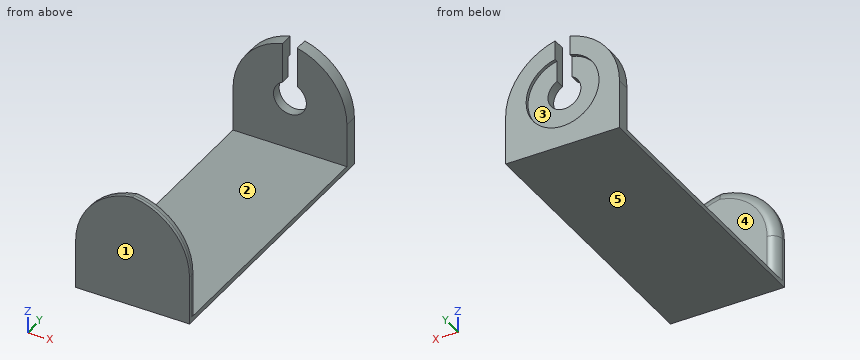
from build123d import *

# Parameters (mm, degrees)
F1_DEPTH    = 17.5
F2_T1_DEPTH = 104
F2_T3_DEPTH = 104
F4_DEPTH    = 1
F5_DEPTH    = 25
F6_R        = 3


# Not quite as in the source:
# - a fillet or chamfer that OpenCascade refuses, or shapes differently, is made with other operations: its cross-section is extruded or revolved along the edge and cut away or added


with BuildPart() as f1:
    # F0 (on Right) → F1 (new body, symmetric)
    with BuildSketch(Plane.YZ):
        Polygon((-44, 35), (-44, 0), (44, 0), (44, 35), (40, 35), (40, 1.5), (-40, 1.5), (-40, 35), align=None)
    extrude(amount=F1_DEPTH, both=True)

    # F2: fillet of radius 20 on 4 edges, made by hand

    # F2_s2 → F2_t1 (cut)
    with BuildSketch(Plane.XZ.offset(-94)):
        with BuildLine():
            ThreePointArc((-2.5, 35), (11.6421356237, 29.1421356237), (17.5, 15))
            Line((17.5, 15), (17.5, 35))
            Line((17.5, 35), (-2.5, 35))
        make_face()
        with BuildLine():
            ThreePointArc((2.5, 35), (-11.6421356237, 29.1421356237), (-17.5, 15))
            Line((-17.5, 15), (-17.5, 35))
            Line((-17.5, 35), (2.5, 35))
        make_face()
    extrude(amount=F2_T1_DEPTH, mode=Mode.SUBTRACT)

    # F2_s4 → F2_t3 (cut)
    with BuildSketch(Plane.XZ.offset(-10)):
        with BuildLine():
            ThreePointArc((2.5, 35), (-11.6421356237, 29.1421356237), (-17.5, 15))
            Line((-17.5, 15), (-17.5, 35))
            Line((-17.5, 35), (2.5, 35))
        make_face()
        with BuildLine():
            ThreePointArc((-2.5, 35), (11.6421356237, 29.1421356237), (17.5, 15))
            Line((17.5, 15), (17.5, 35))
            Line((17.5, 35), (-2.5, 35))
        make_face()
    extrude(amount=F2_T3_DEPTH, mode=Mode.SUBTRACT)

    # F3 (on face) → F4 (cut)
    with BuildSketch(Plane(origin=(0, 44, 0), x_dir=(-1, 0, 0), z_dir=(0, 1, 0))):
        with BuildLine():
            Line((2.25, 22.0293655688), (2.25, 28.4799718057))
            ThreePointArc((2.25, 28.4799718057), (0, 28.7083037466), (-2.25, 28.4799718057))
            Line((-2.25, 28.4799718057), (-2.25, 22.0293655688))
            ThreePointArc((-2.25, 22.0293655688), (0, 12.4583037466), (2.25, 22.0293655688))
        make_face()
        with BuildLine():
            ThreePointArc((-2.25, 28.4799718057), (-7.0795480082, 8.8295941651), (11.2, 17.5083037466))
            ThreePointArc((11.2, 17.5083037466), (8.6787095815, 24.5878517548), (2.25, 28.4799718057))
            Line((2.25, 28.4799718057), (2.25, 22.0293655688))
            ThreePointArc((2.25, 22.0293655688), (0, 12.4583037466), (-2.25, 22.0293655688))
            Line((-2.25, 22.0293655688), (-2.25, 28.4799718057))
        make_face()
    extrude(amount=-F4_DEPTH, mode=Mode.SUBTRACT)

    # F3 (on face) → F5 (cut)
    with BuildSketch(Plane(origin=(0, 44, 0), x_dir=(-1, 0, 0), z_dir=(0, 1, 0))):
        with BuildLine():
            Line((2.25, 22.0293655688), (2.25, 28.4799718057))
            ThreePointArc((2.25, 28.4799718057), (0, 28.7083037466), (-2.25, 28.4799718057))
            Line((-2.25, 28.4799718057), (-2.25, 22.0293655688))
            ThreePointArc((-2.25, 22.0293655688), (0, 12.4583037466), (2.25, 22.0293655688))
        make_face()
        with BuildLine():
            ThreePointArc((-2.25, 28.4799718057), (0, 28.7083037466), (2.25, 28.4799718057))
            Line((2.25, 28.4799718057), (2.25, 34.4277507705))
            ThreePointArc((2.25, 34.4277507705), (1.1309449156, 34.6676444705), (0, 34.843134833))
            ThreePointArc((0, 34.843134833), (-1.1309449156, 34.6676444705), (-2.25, 34.4277507705))
            Line((-2.25, 34.4277507705), (-2.25, 28.4799718057))
        make_face()
    extrude(amount=-F5_DEPTH, mode=Mode.SUBTRACT)

    # F6
    f6_edges = [f1.edges().sort_by_distance(p)[0] for p in [
        (17.5, -40, 8.25),
        (-17.5, -40, 8.25),
    ]]
    fillet(f6_edges, radius=F6_R)


solid = f1.part
Verification items for the finished model (mm, model axes). Face numbers are marked on the shaded views. A direction names the side the tool comes from. Give positions to 0.01 mm unless a question says otherwise; leave off trailing zeros. Write each loop counter-clockwise with the first axis right and the second up, starting at its lowest first coordinate (ties: lowest second). Pieces come first, ordered by that corner, then holes.
(1) Cross-section at C-C (z = 25.5). State how many separate pieces and enclosed holes the cut face has, plus the area to 3 significant figures.
(2) Mould release check, pull along Y, two halves, no side actions. Record for the marked faces 1, 2 and 3: +Y half, -Y half, draft (parallel to the pull), parting line (faces both ways), or undercut.
(3) Cross-section at A-A (z = 4.5). Enter the section's corners in (x, y), plus the area to 3 significant figures.
(4) Cross-section at B-B (y = 16). Enter the section's corners in (x, z).
(5) Access from +Z, -Z, +X, -X, +Y, -Y to the whole of each face (thin tool, end or side, straight path). Record for the marked faces 4 and 5.
(6) Gauge pin test, flat ends, axial feed: pin 1 (4 mm diameter, centred on x = 0, z = 12, fed in from +Y); pin 2 (4.5 mm diameter, centred on y = 41.5, z = 25.5, fed in from -X); pin 3 (2 mm diameter, centred on y = 42.5, z = 25.5, fed in from +X). Record the tip position at first contact, or that the pin passes through.
(7) Material ranges on line 1 (Y direction, x = 9.5, z = 10.5); line 2 (Y direction, x = -1.5, z = 7.5); line 3 (Z direction, x = 10, y = 2), recorded low to high.
Worked out:
1. separate pieces: 3
1. enclosed holes: 0
1. area: 199 mm2
2. face 1: -Y half
2. face 2: undercut
2. face 3: +Y half
3. outline: (-17.5, -44) - (17.5, -44) - (17.5, -43) arc R3 ccw to (14.5, -40) - (-14.5, -40) arc R3 ccw to (-17.5, -43) - close; (-17.5, 40) - (17.5, 40) - (17.5, 44) - (-17.5, 44) - close
3. area: 276 mm2
4. outline: (-17.5, 0) - (17.5, 0) - (17.5, 1.5) - (-17.5, 1.5) - close
5. face 4: +Z, +X, -X
5. face 5: -Z, +X, -X, +Y, -Y
6. pin 1: stops at y = 43
6. pin 2: stops at x = -15.72
6. pin 3: stops at x = 15.1
7. line 1: y = -44 to -40, 40 to 44
7. line 2: y = -44 to -40, 40 to 43
7. line 3: z = 0 to 1.5
